Can you work these out from the model? Positions are in its coordinate system, mm. Give positions to 0.01 mm unless a question says otherwise; leave off trailing zeros. Loops run counter-clockwise (first coordinate to the right, second up) from the corner with the lowest first, then second, coordinate; pieces in that order, holes last.
from build123d import *

# Parameters (mm, degrees)
F0_W     = 54
F0_H     = 82
F0_R     = 2.5
F0_R_2   = 8
F1_DEPTH = 5
F2_R     = 1
F3_R     = 8
F4_DEPTH = 25
F5_DEPTH = 2


with BuildPart() as f1:
    # F0 (on Top) → F1 (new body)
    with BuildSketch(Plane.XY):
        Rectangle(F0_W, F0_H)
        with Locations((-19, -33)):
            Circle(F0_R, mode=Mode.SUBTRACT)
        with Locations((0, -26)):
            Circle(F0_R_2, mode=Mode.SUBTRACT)
        with Locations((19, -33)):
            Circle(F0_R, mode=Mode.SUBTRACT)
        with Locations((-19, 0)):
            Circle(F0_R, mode=Mode.SUBTRACT)
        with Locations((-19, 33)):
            Circle(F0_R, mode=Mode.SUBTRACT)
        with Locations((19, 0)):
            Circle(F0_R, mode=Mode.SUBTRACT)
        with Locations((0, 26)):
            Circle(F0_R_2, mode=Mode.SUBTRACT)
        with Locations((19, 33)):
            Circle(F0_R, mode=Mode.SUBTRACT)
    extrude(amount=F1_DEPTH)

    # F2
    f2_edges = [f1.edges().sort_by_distance(p)[0] for p in [
        (27, -41, 2.5),
        (-27, -41, 2.5),
        (-27, 41, 2.5),
        (27, 41, 2.5),
    ]]
    fillet(f2_edges, radius=F2_R)

    # F3 (on face) → F4 (cut)
    with BuildSketch(Plane.XY.offset(5)):
        Circle(F3_R)
    extrude(amount=-F4_DEPTH, mode=Mode.SUBTRACT)

    # F5 (cut): a face of the model
    f5_faces = [f1.faces().sort_by_distance(p)[0] for p in [
        (26.0181649833, 0, 5),
    ]]
    extrude(f5_faces, amount=-F5_DEPTH, mode=Mode.SUBTRACT)


solid = f1.part
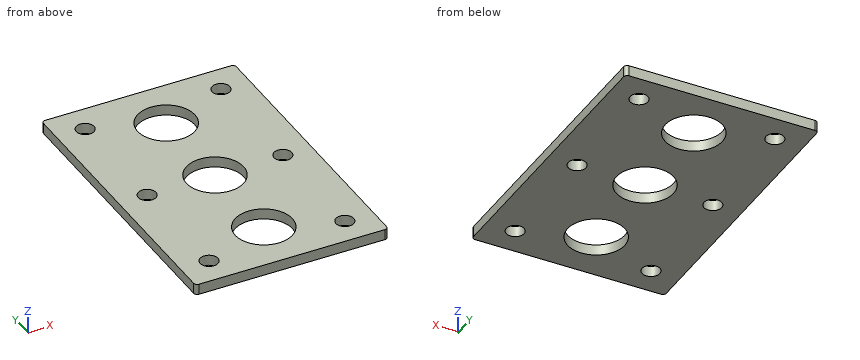
(1) Suppose I cut it at D-D on z = 2. Give the number of separate pieces and of enclosed holes in the cut face, plus the area to 3 significant figures.
Returned:
separate pieces: 1
enclosed holes: 9
area: 3,710 mm2
(2) Please list where these lines run through material, in increasing order: probe 1 along Y at (x, z) = (0, 1); probe 2 along Y at (x, z) = (-19, 0.75); probe 3 along X at (y, z) = (2, 0.95).
Returned:
probe 1: y = -41 to -34, -18 to -8, 8 to 18, 34 to 41
probe 2: y = -41 to -35.5, -30.5 to -2.5, 2.5 to 30.5, 35.5 to 41
probe 3: x = -27 to -20.5, -17.5 to -7.75, 7.75 to 17.5, 20.5 to 27
(3) Suppose I cut it at A-A on y = 0. List the corners of the cut face in (x, z) for me, plus the area to 3 significant figures.
Returned:
outline: (-27, 0) - (-21.5, 0) - (-21.5, 3) - (-27, 3) - close; (-16.5, 0) - (-8, 0) - (-8, 3) - (-16.5, 3) - close; (8, 0) - (16.5, 0) - (16.5, 3) - (8, 3) - close; (21.5, 0) - (27, 0) - (27, 3) - (21.5, 3) - close
area: 84.0 mm2
(4) Suppose I cut it at B-B on y = 26. List the corners of the cut face in (x, z) for me, plus the area to 3 significant figures.
Returned:
outline: (-27, 0) - (-8, 0) - (-8, 3) - (-27, 3) - close; (8, 0) - (27, 0) - (27, 3) - (8, 3) - close
area: 114 mm2
(5) Suppose I cut it at C-C on x = 0. List the corners of the cut face in (y, z) for me, plus the area to 3 significant figures.
Returned:
outline: (-41, 0) - (-34, 0) - (-34, 3) - (-41, 3) - close; (-18, 0) - (-8, 0) - (-8, 3) - (-18, 3) - close; (8, 0) - (18, 0) - (18, 3) - (8, 3) - close; (34, 0) - (41, 0) - (41, 3) - (34, 3) - close
area: 102 mm2
